Geometry: final body of the model. Coordinates: model frame, mm. Face numbers are marked on the shaded views. A direction names the side the tool comes from. Round coordinates to 2 decimals unless told otherwise and drop trailing zeros. Loops run counter-clockwise (first coordinate to the right, second up) from the corner with the lowest first, then second, coordinate; pieces in that order, holes last. Notation, with made-up numbers: (18, -5) - (59, -5) arc R23 ccw to (59, 3) - close; hole circle Ø1 at (75.5, -23). An arc over 180 degrees is marked (long way). Return JSON: item names as keys, results as strings. Group by question number.
1. Set-up query: the marked faces 1 and 2. Return all of +Z, -Z, +X, -X, +Y, -Y with unobstructed straight access to the full face (end or side cutting, diameter ignored); none if empty.
2. Section A-A on y = -26. Return loops of the section in (x, z) (1 decimal).
3. Material intervals for probe 1 along Z at (x, y) = (-91, -39.5); probe 2 along Y at (x, z) = (-7, 13); probe 3 along Z at (x, y) = (37.5, -9), sorted ascending.
4. Section C-C on x = 69.5. Return loops of the section in (y, z) (3 decimals), and give its area (3 significant figures).
5. Section B-B on x = -14. Return loops of the section in (y, z) (3 decimals).
6. Section D-D on z = 8. Return loops of the section in (x, y) (3 decimals), and give its area (3 significant figures).
7. First-contact query: pin 1 Ø3 at (x, z) = (90.5, 39.5) entering from -Y; pin 2 Ø11.5 at (x, y) = (10, -36) entering from -Z; pin 3 Ø1.6 at (x, y) = (-1, -1) entering from -Z. Flat tips, straight axial feed; report the tip coordinate or a pass-through.
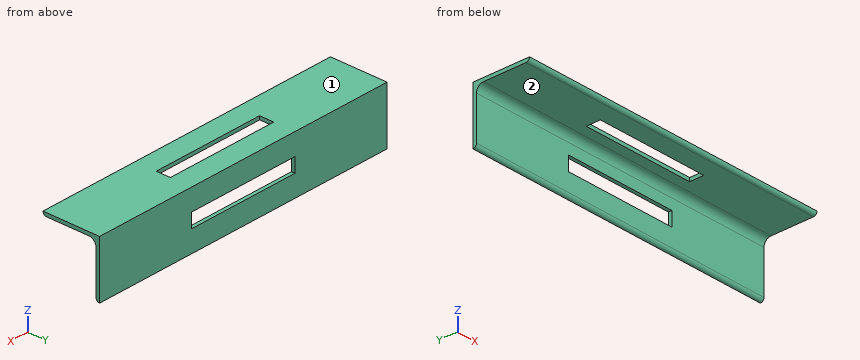
from build123d import *

# Parameters (mm, degrees)
F1_DEPTH      = 282.575
F4_W          = 101.6
F4_H          = 12.7
F5_DEPTH      = 25.4
F5_DEPTH_BACK = 25.4
F3_W          = 101.6
F3_H          = 12.7
F6_DEPTH      = 25.4
F6_DEPTH_BACK = 25.4


with BuildPart() as f1:
    # F0 (on Right) → F1 (new body)
    with BuildSketch(Plane.YZ):
        with BuildLine():
            Line((-0.102489, -7.189187), (0, -7.192553))
            Line((0, -7.192553), (0, 43.607447))
            Line((0, 43.607447), (-50.8, 43.607447))
            ThreePointArc((-50.8, 43.607447), (-49.870064, 41.362383), (-47.625, 40.432447))
            Line((-47.625, 40.432447), (-9.52329, 40.432447))
            ThreePointArc((-9.52329, 40.432447), (-5.033162, 38.572575), (-3.17329, 34.082447))
            Line((-3.17329, 34.082447), (-3.17329, -4.015898))
            ThreePointArc((-3.17329, -4.015898), (-2.279896, -6.223814), (-0.102489, -7.189187))
        make_face()
    extrude(amount=F1_DEPTH)


with BuildPart() as f1_1:
    # F2: moved
    add(f1.part.moved(Location((-137.16, 0, 1.524))))

    # F4 (on face) → F5 (cut, two sides)
    with BuildSketch(Plane.XZ.offset(3.17329)) as f5_sk:
        with Locations((4.1275, 19.737222)):
            Rectangle(F4_W, F4_H)
    extrude(amount=-F5_DEPTH, mode=Mode.SUBTRACT)
    extrude(f5_sk.sketch, amount=-F5_DEPTH_BACK, mode=Mode.SUBTRACT)

    # F3 (on face) → F6 (cut, two sides)
    with BuildSketch(Plane.XY.offset(45.131447)) as f6_sk:
        with Locations((4.1275, -25.4)):
            Rectangle(F3_W, F3_H)
    extrude(amount=-F6_DEPTH, mode=Mode.SUBTRACT)
    extrude(f6_sk.sketch, amount=-F6_DEPTH_BACK, mode=Mode.SUBTRACT)


solid = f1_1.part
Taken from the geometry:
{
 "1": {"face 1": "+Z, +X, -X, +Y, -Y", "face 2": "-Z, +X, -X, -Y"},
 "2": {"outline": "(-137.2, 42) - (-46.7, 42) - (-46.7, 45.1) - (-137.2, 45.1) - close; (54.9, 42) - (145.4, 42) - (145.4, 45.1) - (54.9, 45.1) - close"},
 "3": {"probe 1": "41.96 to 45.13", "probe 2": "-3.17 to 0", "probe 3": "41.93 to 45.13"},
 "4": {"outline": "(-50.8, 45.131) arc R3.175 ccw to (-47.625, 41.956) - (-9.523, 41.956) arc R6.35 cw to (-3.173, 35.606) - (-3.173, -2.492) arc R3.175 ccw to (-0.102, -5.665) - (0, -5.669) - (0, 45.131) - close", "area": "317 mm2"},
 "5": {"outline": "(-50.8, 45.131) arc R3.175 ccw to (-47.625, 41.956) - (-31.75, 41.956) - (-31.75, 45.131) - close; (-19.05, 41.956) - (-9.523, 41.956) arc R6.35 cw to (-3.173, 35.606) - (-3.173, 26.087) - (0, 26.087) - (0, 45.131) - (-19.05, 45.131) - close; (-3.173, -2.492) arc R3.175 ccw to (-0.102, -5.665) - (0, -5.669) - (0, 13.387) - (-3.173, 13.387) - close"},
 "6": {"outline": "(-137.16, -3.173) - (145.415, -3.173) - (145.415, 0) - (-137.16, 0) - close", "area": "897 mm2"},
 "7": {"pin 1": "y = -6.17", "pin 2": "z = 41.96", "pin 3": "z = -5.66"}
}
